Source: CAD feature listing. Evaluate the final solid. Frame: model axes, mm. Face numbers are marked on the shaded views. A direction names the side the tool comes from. Give positions to 0.01 mm unless a question says otherwise; leave off trailing zeros. Order: outer loops, then holes, each group sorted by start corner. A loop starts at its lowest first (then second) coordinate and runs counter-clockwise, first axis right, second up. Notation, with made-up numbers: M -17.75,21 L -13.75,21 A14 cw -13.75,46 Z; hole C 71,-27.5 d1. An arc over 180 degrees is marked long. Answer as a JSON object with one key per item and string values. Group by question number.
1. Section query D-D (y = -2.25). Output: boundary loops of the cut face in (x, z).
2. Material intervals for L1, parallel to X at y = 2.5, z = 8.75; L2, parallel to Y at x = 0, z = 5.75; L3, parallel to X at y = 2.25, z = 11, sorted ascending. Write a range as [from, to].
3. Set-up query: the marked faces 4, 5 and 6. Return all of +Z, -Z, +X, -X, +Y, -Y with unobstructed straight access to the full face (end or side cutting, diameter ignored); none if empty.
4. Section query B-B (y = 0.75). Output: boundary loops of the cut face in (x, z), plus the area to 3 significant figures.
5. Pull-direction query (Y, two-part tool) for the marked faces 1, 2 and 3; classes: +Y half, -Y half, draft (parallel to the pull), parting line (faces both ways), or undercut.
6. Section query A-A (z = 8.5). Output: boundary loops of the cut face in (x, y) (3 decimals), plus the area to 3 significant figures.
7. Section query C-C (x = 0.75). Output: boundary loops of the cut face in (y, z), plus the area to 3 significant figures.
8. Pin query (flat end, axial travel): P1, Ø3, axis at y = 3, z = 3.5, coming from the +X side; P2, Ø2, axis at y = -3, z = 5, coming from the -X side; P3, Ø1.5, axis at y = -1, z = 3, coming from the -X side. Return the tip coordinate at first contact, or that it passes through.
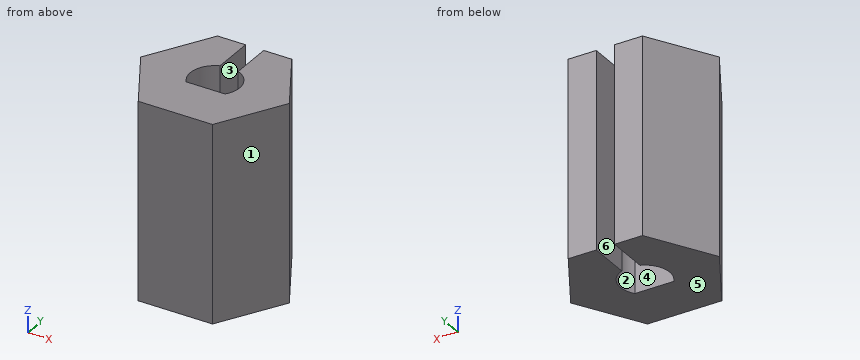
from build123d import *

# Parameters (mm, degrees)
BOSS_EXTRUDE1_DEPTH = 13


with BuildPart() as part:
    # Sketch1 → Boss-Extrude1 (new body)
    with BuildSketch(Plane.XY):
        with BuildLine():
            Line((1.280868846, -1), (-1.280868846, -1))
            ThreePointArc((-1.280868846, -1), (-1.568330344, 0.425399731), (-0.6, 1.510173831))
            Line((-0.6, 1.510173831), (-0.6, 4.243524479))
            Line((-0.6, 4.243524479), (-2.45, 4.243524479))
            Line((-2.45, 4.243524479), (-4.9, 0))
            Line((-4.9, 0), (-2.45, -4.243524479))
            Line((-2.45, -4.243524479), (2.45, -4.243524479))
            Line((2.45, -4.243524479), (4.9, 0))
            Line((4.9, 0), (2.45, 4.243524479))
            Line((2.45, 4.243524479), (0.6, 4.243524479))
            Line((0.6, 4.243524479), (0.6, 1.510173831))
            ThreePointArc((0.6, 1.510173831), (1.568330344, 0.425399731), (1.280868846, -1))
        make_face()
    extrude(amount=BOSS_EXTRUDE1_DEPTH)


solid = part.part
Answer sheet:
{
 "1": {"outline": "M -3.6,0 L 3.6,0 L 3.6,13 L -3.6,13 Z"},
 "2": {"L1": "[-3.46, -0.6], [0.6, 3.46]", "L2": "[-4.24, -1]", "L3": "[-3.6, -0.6], [0.6, 3.6]"},
 "3": {"face 4": "+Z, -Z", "face 5": "-Z, +X, -X, +Y, -Y", "face 6": "+Z, -Z, +Y"},
 "4": {"outline": "M -4.47,0 L -1.44,0 L -1.44,13 L -4.47,13 Z; M 1.44,0 L 4.47,0 L 4.47,13 L 1.44,13 Z", "area": "78.7 mm^2"},
 "5": {"face 1": "-Y half", "face 2": "undercut", "face 3": "draft"},
 "6": {"outline": "M -4.9,0 L -2.45,-4.244 L 2.45,-4.244 L 4.9,0 L 2.45,4.244 L 0.6,4.244 L 0.6,1.51 A1.625 cw 1.281,-1 L -1.281,-1 A1.625 cw -0.6,1.51 L -0.6,4.244 L -2.45,4.244 Z", "area": "52.0 mm^2"},
 "7": {"outline": "M -4.24,0 L -1,0 L -1,13 L -4.24,13 Z; M 1.44,0 L 4.24,0 L 4.24,13 L 1.44,13 Z", "area": "78.6 mm^2"},
 "8": {"P1": "x = 4.03", "P2": "x = -3.75", "P3": "x = -4.76"}
}
